from build123d import *

# Parameters (mm, degrees)
SKETCH_1_R          = 20
EXTRUDE_1_DEPTH     = 2
SKETCH_2_R          = 10
EXTRUDE_2_DEPTH     = 4
SKETCH_3_R          = 1
EXTRUDE_3_DEPTH     = 4
CUT_EXTRUDE_1_DEPTH = 8


with BuildPart() as part:
    # 草图1 → 凸台-拉伸1 (new body)
    with BuildSketch(Plane.XY):
        Circle(SKETCH_1_R)
    extrude_1 = extrude(amount=EXTRUDE_1_DEPTH)

    # 草图2 → 凸台-拉伸2 (add)
    with BuildSketch(Plane.XY.offset(2)):
        Circle(SKETCH_2_R)
    extrude(amount=EXTRUDE_2_DEPTH)

    # 草图3 → 凸台-拉伸3 (add)
    with BuildSketch(Plane.XY.offset(2)):
        with Locations((0.039532003, 11.681707008)):
            Circle(SKETCH_3_R)
    extrude(amount=EXTRUDE_3_DEPTH)

    # 镜向2: 凸台-拉伸1 across plane
    add(extrude_1.mirror(Plane.XY.offset(4)))

    # 草图4 → 切除-拉伸1 (cut)
    with BuildSketch(Plane.XY.offset(8)):
        with BuildLine():
            Line((-1.356465997, -2.1), (1.356465997, -2.1))
            ThreePointArc((1.356465997, -2.1), (0, 2.5), (-1.356465997, -2.1))
        make_face()
    extrude(amount=-CUT_EXTRUDE_1_DEPTH, mode=Mode.SUBTRACT)


solid = part.part
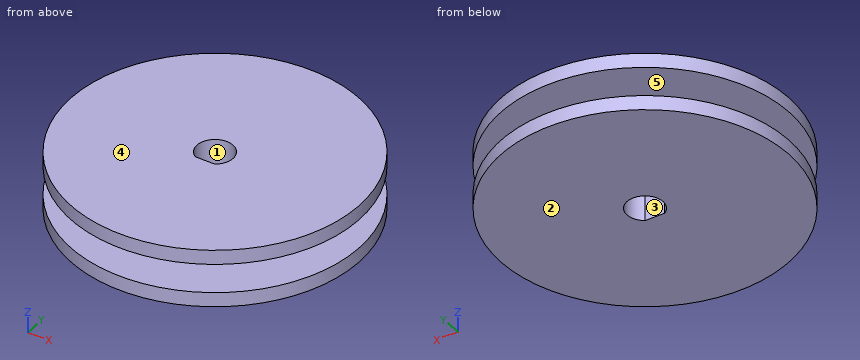
Geometry: final body of the model. Coordinates: model frame, mm. Face numbers are marked on the shaded views. A direction names the side the tool comes from. Give positions to 0.01 mm unless a question says otherwise; leave off trailing zeros. Write each loop counter-clockwise with the first axis right and the second up, starting at its lowest first coordinate (ties: lowest second). Pieces come first, ordered by that corner, then holes. Notation, with made-up numbers: (80.5, -27.75) -> (123.5, -27.75) arc R19 ccw to (123.5, -21.75) -> close; hole circle Ø1 at (-6, 88). An arc over 180 degrees is marked (long way). Answer as a JSON object with one key per item and string values.
1. Cut plane C-C on x = 14. Output: boundary loops of the cut face in (y, z).
Ans:
{"outline": "(-14.28, 0) -> (14.28, 0) -> (14.28, 2) -> (-14.28, 2) -> close; (-14.28, 6) -> (14.28, 6) -> (14.28, 8) -> (-14.28, 8) -> close"}
2. Cut plane A-A on y = 0. Output: boundary loops of the cut face in (x, z).
Ans:
{"outline": "(-20, 0) -> (-2.5, 0) -> (-2.5, 8) -> (-20, 8) -> (-20, 6) -> (-10, 6) -> (-10, 2) -> (-20, 2) -> close; (2.5, 0) -> (20, 0) -> (20, 2) -> (10, 2) -> (10, 6) -> (20, 6) -> (20, 8) -> (2.5, 8) -> close"}
3. Mould query, pull axis Y, two halves, no side actions, for the marked faces 1 and 2. Classes: pulls with the +Y half, pulls with the -Y half, needs draft (parallel to the pull), parting line crosses it, or undercut.
Ans:
{"face 1": "undercut", "face 2": "needs draft"}
4. Ray query, probe 1 along Z at (x, y) = (15, -5.5); probe 2 along Y at (x, z) = (15.5, 7); probe 3 along Y at (x, z) = (4, 5.75). Return the intervals inside material, ascending. Write a range as from..to.
Ans:
{"probe 1": "z = 0..2, 6..8", "probe 2": "y = -12.64..12.64", "probe 3": "y = -9.17..9.17"}
5. Contact query for flat-ended pins moving along their axis: pin 1 (1 mm diameter, centred on y = -2, z = 4, fed in from +X); pin 2 (2 mm diameter, centred on y = -4, z = 2.5, fed in from +X); pin 3 (3 mm diameter, centred on y = -5.5, z = 2.5, fed in from +X); pin 4 (4 mm diameter, centred on x = 0, y = 0, fed in from +Z). Output: stop coordinate, or through.
Ans:
{"pin 1": "stops at x = 9.89", "pin 2": "stops at x = 19.75", "pin 3": "stops at x = 19.58", "pin 4": "passes through"}
6. Access query for the marked faces 3, 4 and 5. Directions: +Z, -Z, +X, -X, +Y, -Y. A direction counts if a zero-diameter tool reaches every point of the face in a straight line with its end or side. Return the directions, or none.
Ans:
{"face 3": "+Z, -Z", "face 4": "+Z, +X, -X, +Y, -Y", "face 5": "none"}
7. Cut plane B-B on x = 0. Output: boundary loops of the cut face in (y, z).
Ans:
{"outline": "(-20, 0) -> (-2.1, 0) -> (-2.1, 8) -> (-20, 8) -> (-20, 6) -> (-10, 6) -> (-10, 2) -> (-20, 2) -> close; (2.5, 0) -> (20, 0) -> (20, 2) -> (12.68, 2) -> (12.68, 6) -> (20, 6) -> (20, 8) -> (2.5, 8) -> close; hole (10, 2) -> (10.68, 2) -> (10.68, 6) -> (10, 6) -> close"}
8. Cut plane D-D on z = 3.25. Output: boundary loops of the cut face in (x, y).
Ans:
{"outline": "circle Ø20 at (0, 0); circle Ø2 at (0.04, 11.68); hole (-1.36, -2.1) -> (1.36, -2.1) arc R2.5 ccw (long way) to start"}
